Verification items for the finished model (mm, model axes). Face numbers are marked on the shaded views. A direction names the side the tool comes from. Give positions to 0.01 mm unless a question says otherwise; leave off trailing zeros. Loops run counter-clockwise (first coordinate to the right, second up) from the corner with the lowest first, then second, coordinate; pieces in that order, holes last. Notation, with made-up numbers: (30.25, 2) - (45.25, 2) arc R22 cw to (45.25, 8) - close; hole circle Ø2 at (-2, 12.5). An arc over 180 degrees is marked (long way). One line per item, written item: value. Start each with the question number.
1. Sectioned sample at B-B (x = -1.5). Record the cut outline in (y, z), plus the area to 3 significant figures.
2. Sectioned sample at D-D (z = 63.5). Record the cut outline in (x, y), plus the area to 3 significant figures.
3. Gauge pin test, flat ends, axial feed: pin 1 (3 mm diameter, centred on x = -7.5, z = 32, fed in from -Y); pin 2 (4 mm diameter, centred on x = 12.5, z = 26.5, fed in from -Y); pin 3 (12 mm diameter, centred on x = 13.5, z = 33.5, fed in from -Y). Record the tip position at first contact, or that the pin passes through.
4. Scan lines: L1, parallel to Z at x = 2.5, y = 6; L2, parallel to Z at x = -19.5, y = 22.5; L3, parallel to Y at x = -1, z = 20.5. Record each from-to range of solid material in increasing order. Write a range as [from, to].
5. Access from +Z, -Z, +X, -X, +Y, -Y to the whole of each face (thin tool, end or side, straight path). Record for the marked faces 1, 2, 3, 4 and 5.
6. Sectioned sample at A-A (z = 36.5). Record the cut outline in (x, y), plus the area to 3 significant figures.
from build123d import *

# Parameters (mm, degrees)
SKETCH1_R           = 25
BOSS_EXTRUDE1_DEPTH = 50
SKETCH2_R           = 5
BOSS_EXTRUDE2_DEPTH = 30
SKETCH3_W           = 50
SKETCH3_H           = 50
BOSS_EXTRUDE3_DEPTH = 10
FILLET1_R           = 5


with BuildPart() as part:
    # Sketch1 → Boss-Extrude1 (new body)
    with BuildSketch(Plane.XY):
        Circle(SKETCH1_R)
    extrude(amount=BOSS_EXTRUDE1_DEPTH)

    # Sketch2 → Boss-Extrude2 (add)
    with BuildSketch(Plane.XY.offset(50)):
        Circle(SKETCH2_R)
    extrude(amount=BOSS_EXTRUDE2_DEPTH)

    # Sketch3 → Boss-Extrude3 (add)
    with BuildSketch(Plane.XY.offset(50)):
        Rectangle(SKETCH3_W, SKETCH3_H)
    extrude(amount=-BOSS_EXTRUDE3_DEPTH)

    # Fillet1
    fillet1_edges = [part.edges().sort_by_distance(p)[0] for p in [
        (25, 25, 45),
        (25, -25, 45),
        (-25, -25, 45),
        (-25, 25, 45),
    ]]
    fillet(fillet1_edges, radius=FILLET1_R)


solid = part.part
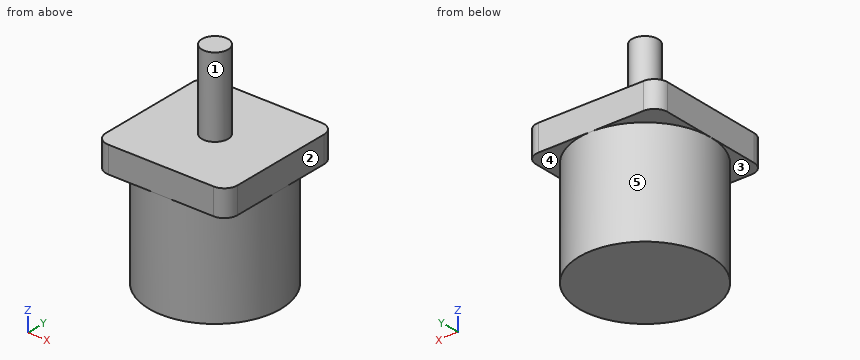
Results are:
1. outline: (-25, 40) - (-24.95, 40) - (-24.95, 0) - (24.95, 0) - (24.95, 40) - (25, 40) - (25, 50) - (4.77, 50) - (4.77, 80) - (-4.77, 80) - (-4.77, 50) - (-25, 50) - close
1. area: 2,780 mm^2
2. outline: circle Ø10 at (0, 0)
2. area: 78.5 mm^2
3. pin 1: stops at y = -24.27
3. pin 2: stops at y = -22.69
3. pin 3: stops at y = -23.85
4. L1: z = [0, 50]
4. L2: z = [40, 50]
4. L3: y = [-24.98, 24.98]
5. face 1: +Z
5. face 2: +Z, -Z, +X, +Y, -Y
5. face 3: -Z, -X, -Y
5. face 4: -Z, +X, +Y
5. face 5: -Z
6. outline: circle Ø50 at (0, 0)
6. area: 1,960 mm^2
